```python
from build123d import *

# Parameters (mm, degrees)
FILLET1_R = 1


with BuildPart() as part:
    # Sketch3 → Revolve1 (revolve)
    with BuildSketch(Plane(origin=(0, 0, 0), x_dir=(1, 0, 0), z_dir=(0, 1, 0))):
        Polygon((6.75, 7.65), (6.75, 5.875), (9.75, 5.875), (12.075, 6.875), (15.875, 6.875), (15.875, 0), (0, 0), (0, 10.15), (2.5, 10.15), (2.5, 7.65), align=None)
    revolve1 = revolve(axis=Axis((0, 0, 0), (0, 0, -1)))

    # Mirror1: Revolve1 across plane
    add(revolve1.mirror(Plane.XY))

    # Fillet1
    fillet1_edges = [part.edges().sort_by_distance(p)[0] for p in [
        (-15.875, 0, 6.875),
        (-15.875, 0, -6.875),
    ]]
    fillet(fillet1_edges, radius=FILLET1_R)


solid = part.part
```
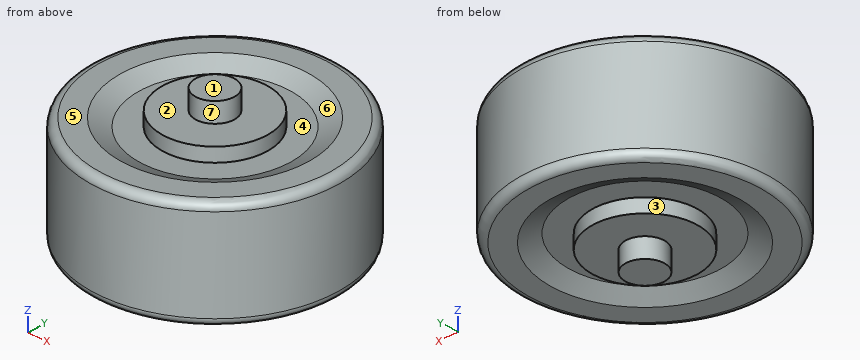
The model under review builds one solid part; all positions refer to its coordinate system, in mm. Face numbers are marked on the shaded views. A direction names the side the tool comes from. Give positions to 0.01 mm unless a question says otherwise; leave off trailing zeros. Use CSV: the item, a comma, the result in double quotes. Start each with the question number.
Q1. To check wall thickness, follow line 1 along Z through (x, y) = (3, -4.5); line 2 along Z through (x, y) = (15, 0); line 3 along X through (y, z) = (-13, 3). State the ranges of each line that lie inside material, in increasing order. Write a range as [from, to].
Q2. The part is to be moulded in two halves that separate along X. For the marked faces 4, 5, 6 and 7, say which applies: +X half, -X half, draft (parallel to the pull), parting line (faces both ways), or undercut.
Q3. Tool access review of the marked faces 1, 2 and 3: name each direction out of +Z, -Z, +X, -X, +Y, -Y from which nothing blocks a thin tool from reaching the whole face with its end or side.
Q4. Clearance check with flat-ended pins moving along their axes: pin 1 Ø6 at (x, y) = (-5, 11) entering from +Z (3 decimals); pin 2 Ø6 at (x, z) = (8, 1) entering from -Y; pin 3 Ø5 at (x, z) = (11.5, 7) entering from -Y. State where each tip first meets the part, or that it passes through.
Outcome:
1,line 1,"z = [-7.65, 7.65]"
1,line 2,"z = [-6.87, 6.87]"
1,line 3,"x = [-9.11, 9.11]"
2,face 4,"undercut"
2,face 5,"draft"
2,face 6,"undercut"
2,face 7,"parting line"
3,face 1,"+Z, +X, -X, +Y, -Y"
3,face 2,"+Z"
3,face 3,"-Z"
4,pin 1,"stops at z = 6.875"
4,pin 2,"stops at y = -15.07"
4,pin 3,"stops at y = -12.93"
